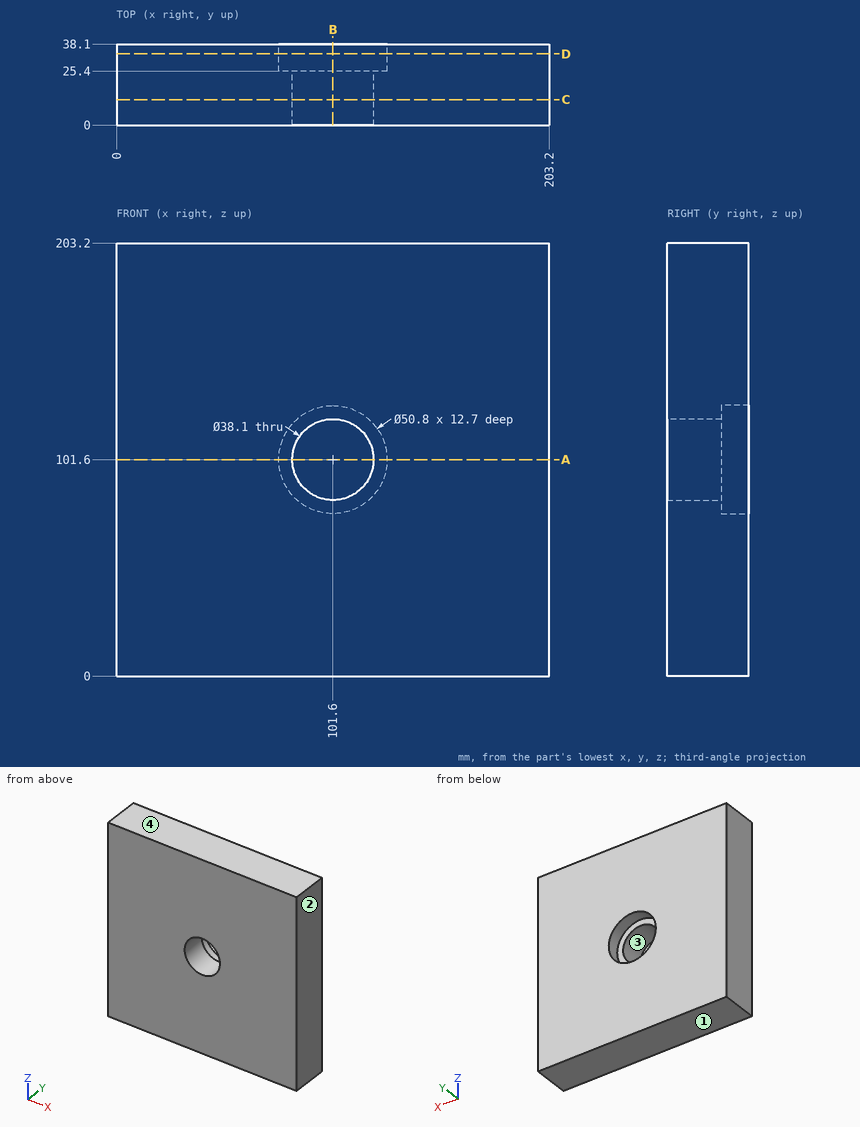
For this review, use the dimensioned drawing (mm, ordinates from the lowest corner) and the shaded views. Give positions to 0.01 mm unless a question says otherwise; leave off trailing zeros. Write each loop counter-clockwise with the first axis right and the second up, starting at its lowest first coordinate (ties: lowest second). Pieces come first, ordered by that corner, then holes. Notation, with made-up numbers: M 1,16.25 L 19,16.25 A11 cw 19,27.25 Z; hole C 10,39 d1. An arc over 180 degrees is marked long. Write item = value, one per line. Start each with the question number.
Q1. We need section A-A (z = 101.6). State the section outline as (x, y) points, plus the area to 3 significant figures.
Q2. Mouldability with a two-part tool opening along Z and no side actions: class the marked faces 1, 2, 3 and 4 as released by +Z, released by -Z, zero draft, split by the parting line, or undercut.
Q3. For line 1 (X direction, y = 12.25, z = 101.6); line 2 (X direction, y = 32.5, z = 101.6); line 3 (Z direction, x = 101, y = 9), list the stretches that pass through material, from the lowest coordinate up.
Q4. We need section D-D (y = 33.5). State the section outline as (x, z) points, plus the area to 3 significant figures.
Q5. We need section C-C (y = 12). State the section outline as (x, z) points, plus the area to 3 significant figures.
Q6. Clearance check with a flat-ended pin moving along its axis: pin 1 (5 mm diameter, centred on y = 31.5, z = 156, fed in from -X). State where the tip first meets the part, or that it passes through.
Q7. We need section B-B (x = 101.6). State the section outline as (y, z) points, plus the area to 3 significant figures.
Result set:
q1.outline = M 0,0 L 82.55,0 L 82.55,25.4 L 76.2,25.4 L 76.2,38.1 L 0,38.1 Z; M 120.65,0 L 203.2,0 L 203.2,38.1 L 127,38.1 L 127,25.4 L 120.65,25.4 Z
q1.area = 6,130 mm2
q2.face_1 = released by -Z
q2.face_2 = zero draft
q2.face_3 = undercut
q2.face_4 = released by +Z
q3.line_1 = 0 to 82.55, 120.65 to 203.2
q3.line_2 = 0 to 76.2, 127 to 203.2
q3.line_3 = 0 to 82.56, 120.64 to 203.2
q4.outline = M 0,0 L 203.2,0 L 203.2,203.2 L 0,203.2 Z; hole C 101.6,101.6 d50.8
q4.area = 39,300 mm2
q5.outline = M 0,0 L 203.2,0 L 203.2,203.2 L 0,203.2 Z; hole C 101.6,101.6 d38.1
q5.area = 40,200 mm2
q6.pin_1 = 0
q7.outline = M 0,0 L 38.1,0 L 38.1,76.2 L 25.4,76.2 L 25.4,82.55 L 0,82.55 Z; M 0,120.65 L 25.4,120.65 L 25.4,127 L 38.1,127 L 38.1,203.2 L 0,203.2 Z
q7.area = 6,130 mm2
